from build123d import *

# Parameters (mm, degrees)
F0_W          = 3.5
F0_H          = 3.5707142143
F0_R          = 1
F1_DEPTH      = 11
F0_W_2        = 5.25
F0_H_2        = 5.25
F2_DEPTH      = 3
F0_R_2        = 4.15
F3_DEPTH      = 8
F3_DEPTH_BACK = 1
F4_DEPTH      = 12
F5_DEPTH      = 4
F6_START      = -9
F0_R_3        = 5
F6_DEPTH      = 3


with BuildPart() as f1:
    # F0 (on Front) → F1 (new body)
    with BuildSketch(Plane.XZ):
        Rectangle(F0_W, F0_H)
        Circle(F0_R, mode=Mode.SUBTRACT)
        Circle(F0_R)
    extrude(amount=F1_DEPTH)

    # F0 (on Front) → F2 (join)
    with BuildSketch(Plane.XZ):
        Rectangle(F0_W_2, F0_H_2)
        with BuildLine():
            ThreePointArc((1.75, 1.7853571071), (2.3048861143, 0.9682458366), (2.5, 0))
            ThreePointArc((2.5, 0), (2.3048861143, -0.9682458366), (1.75, -1.7853571071))
            ThreePointArc((1.75, -1.7853571071), (0, -2.5), (-1.75, -1.7853571071))
            ThreePointArc((-1.75, -1.7853571071), (-2.5, 0), (-1.75, 1.7853571071))
            ThreePointArc((-1.75, 1.7853571071), (0, 2.5), (1.75, 1.7853571071))
        make_face(mode=Mode.SUBTRACT)
        with BuildLine():
            Line((-1.75, -1.7853571071), (-1.75, 1.7853571071))
            ThreePointArc((-1.75, 1.7853571071), (-2.5, 0), (-1.75, -1.7853571071))
        make_face()
        with BuildLine():
            ThreePointArc((1.75, -1.7853571071), (2.3048861143, -0.9682458366), (2.5, 0))
            ThreePointArc((2.5, 0), (2.3048861143, 0.9682458366), (1.75, 1.7853571071))
            Line((1.75, 1.7853571071), (1.75, -1.7853571071))
        make_face()
        with BuildLine():
            ThreePointArc((-1.75, -1.7853571071), (0, -2.5), (1.75, -1.7853571071))
            Line((1.75, -1.7853571071), (-1.75, -1.7853571071))
        make_face()
        with BuildLine():
            Line((-1.75, 1.7853571071), (1.75, 1.7853571071))
            ThreePointArc((1.75, 1.7853571071), (0, 2.5), (-1.75, 1.7853571071))
        make_face()
    extrude(amount=F2_DEPTH)

    # F0 (on Front) → F3 (join, two sides)
    with BuildSketch(Plane.XZ) as f3_sk:
        Circle(F0_R_2)
        Rectangle(F0_W_2, F0_H_2, mode=Mode.SUBTRACT)
    extrude(amount=-F3_DEPTH)
    extrude(f3_sk.sketch, amount=F3_DEPTH_BACK)

    # F0 (on Front) → F4 (join)
    with BuildSketch(Plane.XZ):
        Rectangle(F0_W_2, F0_H_2)
        with BuildLine():
            ThreePointArc((1.75, 1.7853571071), (2.3048861143, 0.9682458366), (2.5, 0))
            ThreePointArc((2.5, 0), (2.3048861143, -0.9682458366), (1.75, -1.7853571071))
            ThreePointArc((1.75, -1.7853571071), (0, -2.5), (-1.75, -1.7853571071))
            ThreePointArc((-1.75, -1.7853571071), (-2.5, 0), (-1.75, 1.7853571071))
            ThreePointArc((-1.75, 1.7853571071), (0, 2.5), (1.75, 1.7853571071))
        make_face(mode=Mode.SUBTRACT)
        Rectangle(F0_W, F0_H)
        Circle(F0_R, mode=Mode.SUBTRACT)
        with BuildLine():
            Line((-1.75, -1.7853571071), (-1.75, 1.7853571071))
            ThreePointArc((-1.75, 1.7853571071), (-2.5, 0), (-1.75, -1.7853571071))
        make_face()
        with BuildLine():
            ThreePointArc((1.75, -1.7853571071), (2.3048861143, -0.9682458366), (2.5, 0))
            ThreePointArc((2.5, 0), (2.3048861143, 0.9682458366), (1.75, 1.7853571071))
            Line((1.75, 1.7853571071), (1.75, -1.7853571071))
        make_face()
        with BuildLine():
            Line((-1.75, 1.7853571071), (1.75, 1.7853571071))
            ThreePointArc((1.75, 1.7853571071), (0, 2.5), (-1.75, 1.7853571071))
        make_face()
        with BuildLine():
            ThreePointArc((-1.75, -1.7853571071), (0, -2.5), (1.75, -1.7853571071))
            Line((1.75, -1.7853571071), (-1.75, -1.7853571071))
        make_face()
    extrude(amount=-F4_DEPTH)

    # F5 (add): a face of the model
    f5_faces = [f1.faces().sort_by_distance(p)[0] for p in [
        (-4.0326202743, 8, 0),
    ]]
    extrude(f5_faces, amount=F5_DEPTH)

    # F0 (on Front) → F6 (join)
    with BuildSketch(Plane.XZ.offset(F6_START)):
        Circle(F0_R_3)
        Circle(F0_R_2, mode=Mode.SUBTRACT)
    extrude(amount=-F6_DEPTH)


solid = f1.part
Could you check a few things on this model? Use its own coordinates, in mm. A direction names the side the tool comes from. Coordinates: 2 decimals unless noted, no trailing zeros. Loops run counter-clockwise (first coordinate to the right, second up) from the corner with the lowest first, then second, coordinate; pieces in that order, holes last.
1. Imagine slicing it at D-D (y = -6.25). Please give me the cut outline in (x, z), and give its area (3 significant figures).
2. Imagine slicing it at B-B (x = 0). Please give me the cut outline in (y, z) (3 decimals).
3. I need wall thicknesses on L1, parallel to Z at x = 0, y = 8; L2, parallel to Y at x = 0.5, z = 0.5; L3, parallel to Z at x = -0.5, y = 8.5. Which ranges of each line are inside material? Lowest first, please.
4. We'd pull the mould along X, two halves only. Please class faces 1 (the face through (0, -7, -1.785)), 2 (the face through (-2.625, -2, 0)), 3 (the face through (2.625, -2, 0)), 4 (the face through (0, 6, -1)): released by +X, released by -X, zero draft, split by the parting line, or undercut.
5. For faces 5 (the face through (0, -2, -2.625)), 6 (the face through (-0.9, 3.93, -4.05)), 7 (the face through (1.75, -7, 0)), 8 (the face through (0, -2, 2.625)), 9 (the face through (0, 0, 0)), which set-ups out of +Z, -Z, +X, -X, +Y, -Y let a thin tool reach every point of the face, with its end or its side?
6. For P1, Ø1.8, axis at y = -7.5, z = 0.5, coming from the -X side; P2, Ø1.8, axis at y = -5.5, z = 0.5, coming from the +X side; P3, Ø1.5, axis at y = -3, z = 3, coming from the -X side (3 decimals), each with a flat end and sliding along its axis, tell me the tip position at first contact or that it passes through.
7. Imagine slicing it at A-A (z = 0). Please give me the cut outline in (x, y) (3 decimals), and give its area (4 significant figures).
8. Imagine slicing it at C-C (y = 0.75). Please give me the cut outline in (x, z), and give its area (3 significant figures).
Computed values:
1. outline: (-1.75, -1.79) - (1.75, -1.79) - (1.75, 1.79) - (-1.75, 1.79) - close
1. area: 12.5 mm2
2. outline: (-11, -1.785) - (-3, -1.785) - (-3, -2.625) - (-1, -2.625) - (-1, -4.15) - (9, -4.15) - (9, -5) - (12, -5) - (12, -1) - (0, -1) - (0, 1) - (12, 1) - (12, 5) - (9, 5) - (9, 4.15) - (-1, 4.15) - (-1, 2.625) - (-3, 2.625) - (-3, 1.785) - (-11, 1.785) - close
3. L1: z = -4.15 to -1, 1 to 4.15
3. L2: y = -11 to 0
3. L3: z = -4.12 to -0.87, 0.87 to 4.12
4. face 1: zero draft
4. face 2: released by -X
4. face 3: released by +X
4. face 4: undercut
5. face 5: -Z, +X, -X, -Y
5. face 6: -Y
5. face 7: +Z, -Z, +X, -Y
5. face 8: +Z, +X, -X, -Y
5. face 9: +Y
6. P1: stops at x = -1.75
6. P2: stops at x = 1.75
6. P3: stops at x = -2.625
7. outline: (-5, 9) - (-4.15, 9) - (-4.15, -1) - (-2.625, -1) - (-2.625, -3) - (-1.75, -3) - (-1.75, -11) - (1.75, -11) - (1.75, -3) - (2.625, -3) - (2.625, -1) - (4.15, -1) - (4.15, 9) - (5, 9) - (5, 12) - (1, 12) - (1, 0) - (-1, 0) - (-1, 12) - (-5, 12) - close
7. area: 127.5 mm2
8. outline: circle Ø8.3 at (0, 0); hole circle Ø2 at (0, 0)
8. area: 51.0 mm2
